from build123d import *

# Parameters (mm, degrees)
BOSS_EXTRUDE1_DEPTH = 12
SKETCH2_R           = 2
SKETCH2_R_2         = 1.5
CUT_EXTRUDE1_DEPTH  = 95.704804524
SKETCH4_W           = 20
SKETCH4_H           = 100
BOSS_EXTRUDE2_DEPTH = 12
FILLET3_R           = 42
FILLET4_R           = 12
SKETCH7_R           = 2
CUT_EXTRUDE3_DEPTH  = 105.732993846
CHAMFER1_SIZE       = 10
FILLET8_R           = 2
CUT_EXTRUDE4_DEPTH  = 105.732993846
CUT_EXTRUDE5_DEPTH  = 105.732993846


with BuildPart() as part:
    # Sketch1 → Boss-Extrude1 (new body)
    with BuildSketch(Plane.XY):
        Polygon((-40, 60), (-25, 60), (-25, 52), (-15, 52), (-15, 0), (-21, 0), (-21, -50), (21, -50), (21, 0), (15, 0), (15, 52), (25, 52), (25, 60), (40, 60), (40, -60), (22, -60), (22, -85), (12, -85), (12, -60), (-12, -60), (-12, -85), (-22, -85), (-22, -60), (-40, -60), align=None)
    extrude(amount=BOSS_EXTRUDE1_DEPTH)

    # Sketch2 → Cut-Extrude1 (cut, through all)
    with BuildSketch(Plane(origin=(0, 0, 0), x_dir=(-1, 0, 0), z_dir=(0, 0, -1))):
        with Locations((-28.5, -32)):
            Circle(SKETCH2_R)
        with Locations((17, -56.5)):
            Circle(SKETCH2_R_2)
        with Locations((28.8, -32)):
            Circle(SKETCH2_R)
        with Locations((-17, -56.5)):
            Circle(SKETCH2_R_2)
    extrude(amount=-CUT_EXTRUDE1_DEPTH, mode=Mode.SUBTRACT)

    # Sketch4 → Boss-Extrude2 (add)
    with BuildSketch(Plane.XY.offset(12)):
        with Locations((-50, 10)):
            Rectangle(SKETCH4_W, SKETCH4_H)
        with Locations((50, 10)):
            Rectangle(SKETCH4_W, SKETCH4_H)
    extrude(amount=-BOSS_EXTRUDE2_DEPTH)

    # Fillet3
    # the kernel refuses this fillet: 42 mm, written as the material it takes off along each edge
    with BuildSketch(Plane(origin=(60, 60, 115.531396204), x_dir=(0, -1, 0), z_dir=(0, 0, -1))) as fillet3_piece_1:
        with BuildLine():
            CenterArc((41.412558482, 42), FILLET3_R, 189.594068227, 80.405931773)
            Line((0, 35), (-0.82825117, 34.86))
            ThreePointArc((-0.82825117, 34.86), (-0.84, 17.5), (-0.84, 0))
            Line((-0.84, 0), (0, -0.84))
            Line((0, -0.84), (41.412558482, -0.84))
            Line((41.412558482, -0.84), (41.412558482, 0))
        make_face()
    extrude(amount=219.062792409, mode=Mode.SUBTRACT)
    with BuildSketch(Plane(origin=(-60, 60, 115.531396204), x_dir=(1, 0, 0), z_dir=(0, 0, -1))) as fillet3_piece_2:
        with BuildLine():
            CenterArc((42, 41.412558482), FILLET3_R, 180, 80.405931773)
            Line((0, 41.412558482), (-0.84, 41.412558482))
            Line((-0.84, 41.412558482), (-0.84, 0))
            Line((-0.84, 0), (0, -0.84))
            ThreePointArc((0, -0.84), (17.5, -0.84), (34.86, -0.82825117))
            Line((34.86, -0.82825117), (35, 0))
        make_face()
    extrude(amount=219.062792409, mode=Mode.SUBTRACT)

    # Fillet4
    fillet4_edges = [part.edges().sort_by_distance(p)[0] for p in [
        (60, -40, 6),
        (-60, -40, 6),
    ]]
    fillet(fillet4_edges, radius=FILLET4_R)

    # Sketch7 → Cut-Extrude3 (cut, through all)
    with BuildSketch(Plane.XY):
        with Locations(Location((-55, -20, 0), (0, 0, 180))):
            Circle(SKETCH7_R)
        with Locations(Location((55, -20, 0), (0, 0, 180))):
            Circle(SKETCH7_R)
        with Locations(Location((-37, -20, 0), (0, 0, 180))):
            Circle(SKETCH7_R)
        with Locations(Location((37, -20, 0), (0, 0, 180))):
            Circle(SKETCH7_R)
    extrude(amount=CUT_EXTRUDE3_DEPTH, mode=Mode.SUBTRACT)

    # Chamfer1
    chamfer1_edges = [part.edges().sort_by_distance(p)[0] for p in [
        (-40, -60, 6),
        (40, -60, 6),
    ]]
    chamfer(chamfer1_edges, length=CHAMFER1_SIZE)

    # Fillet8
    fillet8_edges = [part.edges().sort_by_distance(p)[0] for p in [
        (-30, -60, 6),
        (-40, -50, 6),
        (30, -60, 6),
        (40, -50, 6),
        (40, -40, 6),
        (-40, -40, 6),
    ]]
    fillet(fillet8_edges, radius=FILLET8_R)

    # Sketch8 → Cut-Extrude4 (cut, through all)
    with BuildSketch(Plane(origin=(0, 0, 0), x_dir=(-1, 0, 0), z_dir=(0, 0, -1))):
        with BuildLine():
            ThreePointArc((-17.964817996, 17.438774634), (-30.770630407, 21.535466224), (-44.214817996, 21.375674028))
            ThreePointArc((-44.214817996, 21.375674028), (-45.841525426, 19.061841075), (-43.527692473, 17.435133644))
            ThreePointArc((-43.527692473, 17.435133644), (-31.363903701, 17.579707536), (-19.777692473, 13.87317705))
            ThreePointArc((-19.777692473, 13.87317705), (-17.088456442, 14.749538603), (-17.964817996, 17.438774634))
        make_face()
        with BuildLine():
            ThreePointArc((17.964817996, 17.438774634), (30.770630407, 21.535466224), (44.214817996, 21.375674028))
            ThreePointArc((44.214817996, 21.375674028), (45.841525426, 19.061841075), (43.527692473, 17.435133644))
            ThreePointArc((43.527692473, 17.435133644), (31.363903701, 17.579707536), (19.777692473, 13.87317705))
            ThreePointArc((19.777692473, 13.87317705), (17.088456442, 14.749538603), (17.964817996, 17.438774634))
        make_face()
    extrude(amount=-CUT_EXTRUDE4_DEPTH, mode=Mode.SUBTRACT)

    # Sketch9 → Cut-Extrude5 (cut, through all)
    with BuildSketch(Plane.XY.offset(12)):
        Polygon((-24, 52), (-20, 52), (-20, 45.2), (-18.25, 45.2), (-18.25, 42), (-25.75, 42), (-25.75, 45.2), (-24, 45.2), align=None)
    cut_extrude5 = extrude(amount=-CUT_EXTRUDE5_DEPTH, mode=Mode.SUBTRACT)

    # Mirror1: Cut-Extrude5 across plane
    add(cut_extrude5.mirror(Plane(origin=(0, 0, 0), x_dir=(0, 0, 1), z_dir=(1, 0, 0))), mode=Mode.SUBTRACT)


solid = part.part
Can you work these out from the model? Positions are in its coordinate system, mm. A direction names the side the tool comes from. Round coordinates to 2 decimals unless told otherwise and drop trailing zeros. Loops run counter-clockwise (first coordinate to the right, second up) from the corner with the lowest first, then second, coordinate; pieces in that order, holes last. Notation, with made-up numbers: (-25.75, -5.75) - (-0.75, -5.75) arc R27 cw to (-0.75, 20.25) - close; hole circle Ø8 at (29, 32.5). An arc over 180 degrees is marked (long way). Use CSV: the item, a comma, the result in double quotes. Start each with the question number.
1) Please list where these lines run through material, in increasing order: probe 1 along X at (y, z) = (-20, 9.5); probe 2 along X at (y, z) = (9, 7.5); probe 3 along Y at (x, z) = (-36, 2). Write a range as [from, to].
2) If we section it at B-B on y = 7.5: Write out the boundary of the cut face in (x, z), plus the area to 3 significant figures.
3) If we section it at A-A on y = -20: Write out the boundary of the cut face in (x, z).
4) If we section it at D-D on x = -55: Write out the boundary of the cut face in (y, z), plus the area to 3 significant figures.
5) For pin 1 Ø1.6 at (y, z) = (43, 7.5) entering from -X; pin 2 Ø3.5 at (y, z) = (49, 4) entering from +X; pin 3 Ø3.5 at (x, z) = (-27.5, 5.5) entering from -Y, each with a flat end and sliding along its axis, tell me the tip position at first contact or that it passes through.
6) For faces 5 (the flat face through (-21, -25, 6)), 6 (the flat face through (-20, 49, 6)), 7 (the flat face through (-40, -46, 6)), which set-ups out of +Z, -Z, +X, -X, +Y, -Y let a thin tool reach every point of the face, with its end or its side?
7) We'd pull the mould along X, two halves only. Please class faces 1 (the flat face through (40, -46, 6)), 2 (the flat face through (-17, -85, 6)), 3 (the flat face through (-35, -55, 6)), 4 (the flat face through (-25, 56, 6)): released by +X, released by -X, zero draft, split by the parting line, or undercut.
8) If we section it at C-C on x = 37: Write out the boundary of the cut face in (y, z), plus the area to 3 significant figures.
Geometry results:
1,probe 1,"x = [-60, -57], [-53, -39], [-35, -21], [21, 35], [39, 53], [57, 60]"
1,probe 2,"x = [-60, -15], [15, 60]"
1,probe 3,"y = [-54, -21.73], [-18.27, 17.99], [21.99, 56.53]"
2,outline,"(-60, 0) - (-15, 0) - (-15, 12) - (-60, 12) - close; (15, 0) - (60, 0) - (60, 12) - (15, 12) - close"
2,area,"1,080 mm2"
3,outline,"(-60, 0) - (-57, 0) - (-57, 12) - (-60, 12) - close; (-53, 0) - (-39, 0) - (-39, 12) - (-53, 12) - close; (-35, 0) - (-21, 0) - (-21, 12) - (-35, 12) - close; (21, 0) - (35, 0) - (35, 12) - (21, 12) - close; (39, 0) - (53, 0) - (53, 12) - (39, 12) - close; (57, 0) - (60, 0) - (60, 12) - (57, 12) - close"
4,outline,"(-37.75, 0) - (-22, 0) - (-22, 12) - (-37.75, 12) - close; (-18, 0) - (38.46, 0) - (38.46, 12) - (-18, 12) - close"
4,area,"867 mm2"
5,pin 1,"stops at x = -52.73"
5,pin 2,"stops at x = 48.7"
5,pin 3,"stops at y = -60"
6,face 5,"+Z, -Z"
6,face 6,"+Z, -Z, +Y"
6,face 7,"+Z, -Z, -X, -Y"
7,face 1,"released by +X"
7,face 2,"zero draft"
7,face 3,"released by -X"
7,face 4,"undercut"
8,outline,"(-53, 0) - (-22, 0) - (-22, 12) - (-53, 12) - close; (-18, 0) - (18, 0) - (18, 12) - (-18, 12) - close; (22, 0) - (56.04, 0) - (56.04, 12) - (22, 12) - close"
8,area,"1,210 mm2"
